Here's how the part is built. I have some questions about the finished solid (model axes, mm). A direction names the side the tool comes from. Give positions to 0.01 mm unless a question says otherwise; leave off trailing zeros. Use one line per item in the form item = value. Start each with the question number.
from build123d import *

# Parameters (mm, degrees)
F_1_32_0_03125_DIAMETER_HOLE1_REACH  = 30.292
F_1_32_0_03125_DIAMETER_HOLE1_BORE_R = 0.396875


with BuildPart() as part:
    # Sketch1 → Revolve1 (revolve)
    with BuildSketch(Plane.XY, mode=Mode.PRIVATE) as revolve1_sk:
        Polygon((-6.2484, 12.6492), (-6.2484, 8.550800018), (-1.073308102, 8.550800018), (-1.073308102, 9.17149847), (0, 9.17149847), (0, 8.550800018), (0, 7.6708), (5.207, 7.6708), (5.207, 11.8745), (3.937, 11.8745), (3.937, 10.6045), (1.4478, 10.6045), (1.4478, 11.8745), (-3.7084, 11.8745), (-3.7084, 12.6492), align=None)
    revolve(revolve1_sk.sketch.rotate(Axis((0, 0, 0), (-1, 0, 0)), 90), axis=Axis((0, 0, 0), (-1, 0, 0)))

    # 1/32 (0.03125) Diameter Hole1 bore → 1/32 (0.03125) Diameter Hole1 (cut, up to next)
    with BuildSketch(Plane(origin=(0, 11.8745, 0), x_dir=(1, 0, 0), z_dir=(0, 1, 0)), mode=Mode.PRIVATE) as f_1_32_0_03125_diameter_hole1_sk1:
        with Locations((-0.536654051, 0)):
            Circle(F_1_32_0_03125_DIAMETER_HOLE1_BORE_R)
    f_1_32_0_03125_diameter_hole1_tool1 = extrude(f_1_32_0_03125_diameter_hole1_sk1.sketch, amount=-F_1_32_0_03125_DIAMETER_HOLE1_REACH, mode=Mode.PRIVATE) & part.part
    add(f_1_32_0_03125_diameter_hole1_tool1.solids().sort_by_distance((-0.536654, 11.8745, 0))[0], mode=Mode.SUBTRACT)

    # Sketch4 → Cut-Revolve3 (revolve, cut)
    with BuildSketch(Plane.XY, mode=Mode.PRIVATE) as cut_revolve3_sk:
        with BuildLine():
            Line((-0.139779051, 11.8745), (0.364997855, 11.8745))
            Line((0.364997855, 11.8745), (0.364997855, 10.450394686))
            Line((0.364997855, 10.450394686), (-1.438305958, 10.450394686))
            Line((-1.438305958, 10.450394686), (-1.438305958, 11.8745))
            Line((-1.438305958, 11.8745), (-0.933529051, 11.8745))
            add(Edge.make_bspline(
                [(-0.139779051, 11.8745), (-0.536654051, 11.861235461), (-0.933529051, 11.8745)],
                knots=[0, 0, 0, 1, 1, 1], degree=2, weights=[0.011477625, 0.0118745, 0.012271375]))
        make_face()
    revolve(cut_revolve3_sk.sketch.rotate(Axis((-6.82117, 0, 0), (1, 0, 0)), 270), axis=Axis((-6.82117, 0, 0), (1, 0, 0)), mode=Mode.SUBTRACT)


with BuildPart() as cut_revolve3_kept_piece:
    # of the separate pieces the step leaves, the one the design keeps (cut_revolve3_pieces_kept)
    add(part.part.solids().sort_by_distance((-6.2484, 0, -12.6492))[0])


solid = cut_revolve3_kept_piece.part
1) Thinking about a two-plate mould opening in Z: for faces 4 (the face through (-5, -4, -12)), 5 (the face through (-0.529, -9.093, 1.194)), 6 (the face through (3.937, -10, 4)), which applies, released by +Z, released by -Z, zero draft, split by the parting line, or undercut?
2) Will these pins go through, and if not, where does the flat tip stop? P1, Ø9, axis at y = 0, z = -3.5, coming from the -X side; P2, Ø6, axis at x = 2.5, z = -7.5, coming from the -Y side; P3, Ø7, axis at y = 1.5, z = -2.5, coming from the +X side; P4, Ø6, axis at x = -3, z = 7.5, coming from the +Y side.
3) Suppose I cut it at C-C, the plane z = 0. State how many separate pieces and enclosed holes the cut face has, and give its area (3 significant figures).
4) Please list where these lines run through material, in increasing order: line 1 (X direction, y = -10.5, z = -2.75) (3 decimals); line 2 (X direction, y = 8, z = 4.25); line 3 (Y direction, x = 1, z = -1).
5) On a 3-axis mill with a long thin cutter (end or side, diameter ignored), from which of +Z, -Z, +X, -X, +Y, -Y can I reach the whole of each face in a straight line? I mean faces 1 (the face through (-3.62, 8.35, 1.85)), 2 (the face through (1.448, -10, -4)), 3 (the face through (4.563, -3.567, -11.326)). Say none if no direction works.
Checks:
q1.face_4 = split by the parting line
q1.face_5 = undercut
q1.face_6 = zero draft
q2.P1 = 0
q2.P2 = -10.91
q2.P3 = through
q2.P4 = 11.79
q3.separate_pieces = 3
q3.enclosed_holes = 0
q3.area = 75.4 mm^2
q4.line_1 = -6.248 to -1.438, 0.365 to 1.448, 3.937 to 5.207
q4.line_2 = -6.25 to -1.07, 0 to 5.21
q4.line_3 = -11.83 to -7.61, 7.61 to 11.83
q5.face_1 = -X
q5.face_2 = none
q5.face_3 = +X
